from build123d import *

# Parameters (mm, degrees)
SKETCH3_W           = 10
SKETCH3_H           = 32
BOSS_EXTRUDE1_DEPTH = 10
SKETCH4_R           = 1.6
CUT_EXTRUDE1_DEPTH  = 106.045434916
CUT_EXTRUDE2_START  = -7
SKETCH4_3_R         = 3
SKETCH4_3_R_2       = 1.6
CUT_EXTRUDE2_DEPTH  = 3
CHAMFER1_SIZE       = 20
CHAMFER1_SIZE2      = 3.526539614
CHAMFER2_SIZE       = 5
CHAMFER3_SIZE       = 17.013845459
CHAMFER3_SIZE_2     = 3
FILLET1_R           = 2


with BuildPart() as part:
    # Sketch3 → Boss-Extrude1 (new, symmetric)
    with BuildSketch(Plane(origin=(37.122691811, 0, 0), x_dir=(0, 0, -1), z_dir=(1, 0, 0))):
        Polygon((50, -69.46065261), (0, -69.46065261), (-10, -69.46065261), (-20, -69.46065261), (-20, -79.46065261), (50, -79.46065261), align=None)
        with Locations((-5, -53.46065261)):
            Rectangle(SKETCH3_W, SKETCH3_H)
    extrude(amount=BOSS_EXTRUDE1_DEPTH, both=True)

    # Sketch4 → Cut-Extrude1 (cut, through all)
    with BuildSketch(Plane(origin=(0, 0, 0), x_dir=(-1, 0, 0), z_dir=(0, 0, -1))):
        with Locations(Location((-37.122691811, -43.96065261, 0), (0, 0, 90))):
            Circle(SKETCH4_R)
        with Locations(Location((-37.122691811, -58.96065261, 0), (0, 0, 90))):
            Circle(SKETCH4_R)
    extrude(amount=-CUT_EXTRUDE1_DEPTH, mode=Mode.SUBTRACT)

    # Sketch4<3> → Cut-Extrude2 (cut)
    # profile 1 of 2: a face of its own
    with BuildSketch(Plane(origin=(0, 0, 0), x_dir=(-1, 0, 0), z_dir=(0, 0, -1)).offset(CUT_EXTRUDE2_START)):
        with Locations(Location((-37.122691811, -43.96065261, 0), (0, 0, 90))):
            Circle(SKETCH4_3_R)
        with Locations(Location((-37.122691811, -43.96065261, 0), (0, 0, 90))):
            Circle(SKETCH4_3_R_2, mode=Mode.SUBTRACT)
    # profile 2 of 2: a face of its own
    with BuildSketch(Plane(origin=(0, 0, 0), x_dir=(-1, 0, 0), z_dir=(0, 0, -1)).offset(CUT_EXTRUDE2_START)):
        with Locations(Location((-37.122691811, -58.96065261, 0), (0, 0, 90))):
            Circle(SKETCH4_3_R)
        with Locations(Location((-37.122691811, -58.96065261, 0), (0, 0, 90))):
            Circle(SKETCH4_3_R_2, mode=Mode.SUBTRACT)
    extrude(amount=-CUT_EXTRUDE2_DEPTH, mode=Mode.SUBTRACT)

    # Chamfer1
    chamfer1_edges = [part.edges().sort_by_distance(p)[0] for p in [
        (37.122691811, -69.46065261, -50),
    ]]
    chamfer1_side = [part.faces().sort_by_distance(p)[0] for p in [
        (37.122691811, -69.46065261, -25),
    ]]
    chamfer(chamfer1_edges, length=CHAMFER1_SIZE, length2=CHAMFER1_SIZE2, reference=chamfer1_side[0])

    # Chamfer2
    chamfer2_edges = [part.edges().sort_by_distance(p)[0] for p in [
        (37.122691811, -69.46065261, 20),
    ]]
    chamfer(chamfer2_edges, length=CHAMFER2_SIZE)

    # Chamfer3
    # the kernel refuses this chamfer: 17.013845459, 3 mm, written as the material it takes off along each edge
    with BuildSketch(Plane(origin=(-17.08844569, -37.46065261, 10), x_dir=(0, -0.9999776716360548, 0.006682531656101368), z_dir=(1, 0, 0))) as chamfer3_piece_1:
        Polygon((CHAMFER3_SIZE * 0.999977671627, CHAMFER3_SIZE * 0.00668253165604), (-CHAMFER3_SIZE_2 * 0.0066825316561, CHAMFER3_SIZE_2 * 0.999977671636), (0, 0), align=None)
    extrude(amount=108.422275002, mode=Mode.SUBTRACT)

    # Fillet1
    fillet1_edges = [part.edges().sort_by_distance(p)[0] for p in [
        (37.122691811, -69.46065261, 10),
        (37.122691811, -69.46065261, -30),
        (37.122691811, -72.987192224, -50),
        (37.122691811, -74.46065261, 20),
        (37.122691811, -69.46065261, 15),
        (37.122691811, -54.474498068, 10),
        (37.122691811, -37.46065261, 7),
    ]]
    fillet(fillet1_edges, radius=FILLET1_R)


solid = part.part
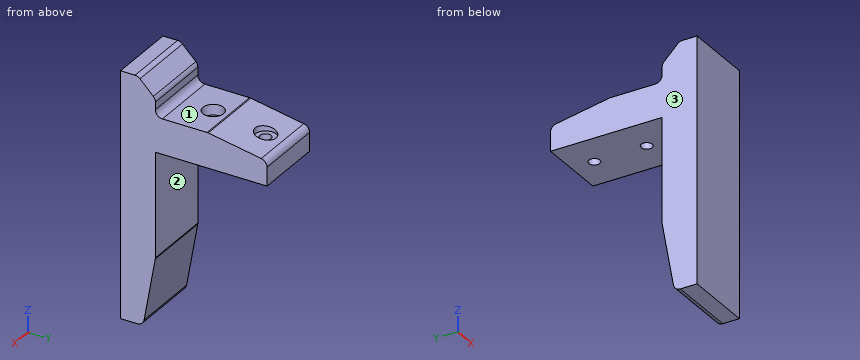
Part model, mm, in its own coordinate system. Face numbers are marked on the shaded views. A direction names the side the tool comes from. Coordinates: 2 decimals unless noted, no trailing zeros. Loops run counter-clockwise (first coordinate to the right, second up) from the corner with the lowest first, then second, coordinate; pieces in that order, holes last. Notation, with made-up numbers: M 35,-11 L 49,-11 A15 ccw 49,-2 Z; hole C -15.75,20 d11. An arc over 180 degrees is marked long. Use a Markdown table: item, result. Add a question column.
Q1. Cut at B-B (x = 45). Write the cut outline in (y, z), and give its area (3 significant figures).
Q2. Probe L1, parallel to Z at x = 38, y = -55.5; L2, parallel to Y at x = 36, z = 12; L3, parallel to Z at x = 35, y = -57. List the from-to ranges inside material, lowest first.
Q3. Pin check, flat tips, straight feed: P1, Ø6, axis at x = 31.5, y = -65.5, coming from the +Z side; P2, Ø3, axis at x = 42, y = -73, coming from the -Z side; P3, Ø1.8, axis at x = 36, y = -44.5, coming from the +Z side. Stop position of each tip, or through.
Q4. Cut at C-C (z = 4.5). Write the cut outline in (x, y), and give its area (3 significant figures).
Q5. Cut at D-D (z = -26.5). Write the cut outline in (x, y).
Q6. Which spindle directions (+Z, -Z, +X, -X, +Y, -Y) get a long thin tool onto all of the face, cutting with end or side? Do the marked faces 1, 2 and 3. Say none if no direction does.
Q7. Cut at A-A (y = -59). Write the cut outline in (x, z).
Worked out:
| question | item | result |
|---|---|---|
| 1 | outline | M -79.46,-50 L -74.67,-50 A2 ccw -72.7,-48.35 L -69.49,-30.17 A2 ccw -69.46,-29.83 L -69.46,0 L -37.46,0 L -37.46,5.32 A2 ccw -39.11,7.29 L -54.3,9.97 A2 ccw -54.65,10 L -67.46,10 A2 cw -69.46,12 L -69.46,14.17 A2 ccw -70.05,15.59 L -73.87,19.41 A2 ccw -75.29,20 L -79.46,20 Z |
| 1 | area | 946 mm2 |
| 2 | L1 | z = 0 to 10 |
| 2 | L2 | y = -79.46 to -69.46 |
| 2 | L3 | z = 0 to 7 |
| 3 | P1 | stops at z = 10.29 |
| 3 | P2 | stops at z = -49.99 |
| 3 | P3 | stops at z = 7 |
| 4 | outline | M 27.12,-79.46 L 47.12,-79.46 L 47.12,-37.46 L 27.12,-37.46 Z; hole C 37.12,-58.96 d3.2; hole C 37.12,-43.96 d3.2 |
| 4 | area | 824 mm2 |
| 5 | outline | M 27.12,-79.46 L 47.12,-79.46 L 47.12,-69.46 L 27.12,-69.46 Z |
| 6 | face 1 | +Z, +X, -X, +Y |
| 6 | face 2 | -Z, +X, -X, +Y |
| 6 | face 3 | +Z, -Z, -X, +Y, -Y |
| 7 | outline | M 27.12,0 L 35.52,0 L 35.52,7 L 34.12,7 L 34.12,10 L 27.12,10 Z; M 38.72,0 L 47.12,0 L 47.12,10 L 40.12,10 L 40.12,7 L 38.72,7 Z |
